Can you work these out from the drawing? Everything is in mm from the part's minimum corner. A direction names the side the tool comes from. Give positions to 0.01 mm unless a question says otherwise; leave off trailing zeros. Loops run counter-clockwise (first coordinate to the right, second up) from the corner with the lowest first, then second, coordinate; pieces in that order, holes last. Notation, with made-up numbers: (85, -5) - (111, -5) arc R26 ccw to (111, 34) - close; hole circle Ø1 at (61, 86). An arc over 180 degrees is marked (long way). Answer in a Markdown table with one row per item. Add a question column.
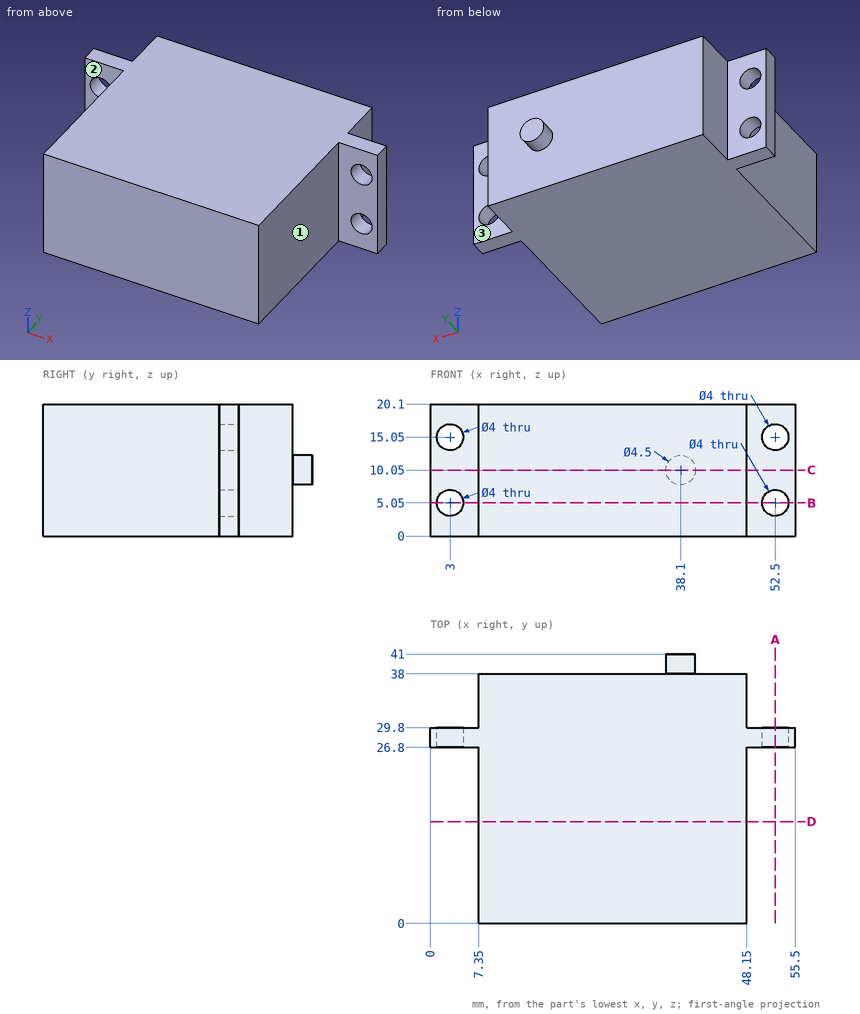
(1) I want a section at C-C on z = 10.05. Please give me the cut outline in (x, y).
(2) I want a section at B-B on z = 5.05. Please give me the cut outline in (x, y), then the cut area to 3 significant figures.
(3) For pin 1 Ø4 at (y, z) = (32.5, 11) entering from +X; pin 2 Ø4 at (y, z) = (34.5, 14.5) entering from -X; pin 3 Ø3.5 at (x, z) = (3, 14.5) entering from -Y; pin 4 Ø3 at (x, z) = (3, 15.05) entering from -Y, each with a flat end and sliding along its axis, tell me the tip position at first contact or that it passes through.
(4) I want a section at A-A on x = 52.5. Please give me the cut outline in (y, z).
(5) I want a section at D-D on y = 15.5. Please give me the cut outline in (x, z).
(6) Please list where these lines run through material, in increasing order: line 1 (X direction, y = 29, z = 15.05); line 2 (Z direction, x = 3, y = 27); line 3 (X direction, y = 29.5, z = 14.5).
(7) On a 3-axis mill with a long thin cutter (end or side, diameter ignored), from which of +Z, -Z, +X, -X, +Y, -Y can I reach the whole of each face in a straight line? I mean the marked faces 1, 2 and 3. Say none if no direction works.
Reported:
| question | item | result |
|---|---|---|
| 1 | outline | (0, 26.8) - (7.35, 26.8) - (7.35, 0) - (48.15, 0) - (48.15, 26.8) - (55.5, 26.8) - (55.5, 29.8) - (48.15, 29.8) - (48.15, 38) - (40.35, 38) - (40.35, 41) - (35.85, 41) - (35.85, 38) - (7.35, 38) - (7.35, 29.8) - (0, 29.8) - close |
| 2 | outline | (0, 26.8) - (1, 26.8) - (1, 29.8) - (0, 29.8) - close; (5, 26.8) - (7.35, 26.8) - (7.35, 0) - (48.15, 0) - (48.15, 26.8) - (50.5, 26.8) - (50.5, 29.8) - (48.15, 29.8) - (48.15, 38) - (7.35, 38) - (7.35, 29.8) - (5, 29.8) - close; (54.5, 26.8) - (55.5, 26.8) - (55.5, 29.8) - (54.5, 29.8) - close |
| 2 | area | 1,570 mm² |
| 3 | pin 1 | x = 48.15 |
| 3 | pin 2 | x = 7.35 |
| 3 | pin 3 | y = 26.8 |
| 3 | pin 4 | through |
| 4 | outline | (26.8, 0) - (29.8, 0) - (29.8, 3.05) - (26.8, 3.05) - close; (26.8, 7.05) - (29.8, 7.05) - (29.8, 13.05) - (26.8, 13.05) - close; (26.8, 17.05) - (29.8, 17.05) - (29.8, 20.1) - (26.8, 20.1) - close |
| 5 | outline | (7.35, 0) - (48.15, 0) - (48.15, 20.1) - (7.35, 20.1) - close |
| 6 | line 1 | 0 to 1, 5 to 50.5, 54.5 to 55.5 |
| 6 | line 2 | 0 to 3.05, 7.05 to 13.05, 17.05 to 20.1 |
| 6 | line 3 | 0 to 1.08, 4.92 to 50.58, 54.42 to 55.5 |
| 7 | face 1 | +Z, -Z, +X, -Y |
| 7 | face 2 | +Z, -Z, -X, -Y |
| 7 | face 3 | +Z, -Z, +X, +Y |
